from build123d import *

# Parameters (mm, degrees)
F1_DEPTH       = 35
F2_SIZE        = 1
F4_D           = 2.5
F4_DEPTH       = 8
F4_TIP         = 0.7510757738
F6_D           = 4.5
F6_CBORE_D     = 8
F6_CBORE_DEPTH = 5
F8_D           = 3.3
F8_DEPTH       = 12
F8_TIP         = 0.9914200214


with BuildPart() as f1:
    # F0 (on Top) → F1 (new body, symmetric)
    with BuildSketch(Plane.XY):
        Polygon((4, 17), (5, 17), (5, 19), (-5, 19), (-5, -19), (5, -19), (5, -17), (4, -17), (4, 0), align=None)
    extrude(amount=F1_DEPTH, both=True)

    # F2
    f2_edges = [f1.edges().sort_by_distance(p)[0] for p in [
        (-5, 19, 0),
        (5, 19, 0),
        (-5, -19, 0),
        (5, -19, 0),
    ]]
    chamfer(f2_edges, length=F2_SIZE)

    # F4
    with Locations(Plane.XY.offset(35)):
        with Locations((0, 13), (0, -13)):
            Hole(F4_D / 2, depth=F4_DEPTH)
            with Locations((0, 0, -(F4_DEPTH + F4_TIP / 2))):  # 118° drill point
                Cone(0, F4_D / 2, F4_TIP, mode=Mode.SUBTRACT)

    # F6 (through all)
    with Locations(Plane(origin=(-5, 0, 0), x_dir=(0, -1, 0), z_dir=(-1, 0, 0))):
        with Locations((-13, 8), (13, 8), (13, -18), (-13, -18)):
            CounterBoreHole(F6_D / 2, F6_CBORE_D / 2, F6_CBORE_DEPTH)

    # F8
    with Locations(Plane(origin=(0, 0, -35), x_dir=(1, 0, 0), z_dir=(0, 0, -1))):
        with Locations((0, 13), (0, 0), (0, -13)):
            Hole(F8_D / 2, depth=F8_DEPTH)
            with Locations((0, 0, -(F8_DEPTH + F8_TIP / 2))):  # 118° drill point
                Cone(0, F8_D / 2, F8_TIP, mode=Mode.SUBTRACT)


solid = f1.part
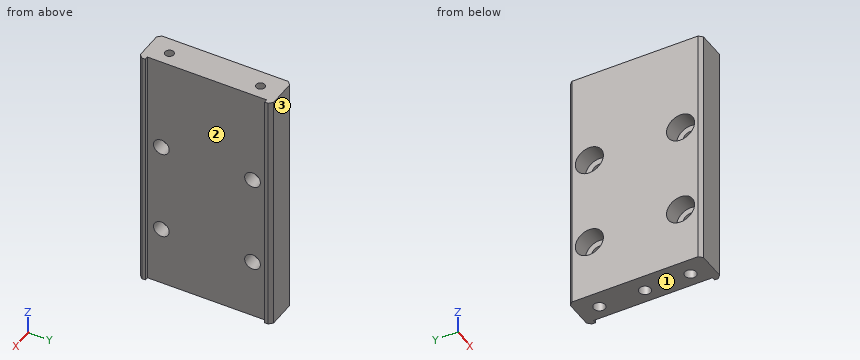
For this review, take the finished solid that the model builds, in its own axes (mm). Face numbers are marked on the shaded views. Round coordinates to 2 decimals unless told otherwise and drop trailing zeros. Write each loop counter-clockwise with the first axis right and the second up, starting at its lowest first coordinate (ties: lowest second). Pieces come first, ordered by that corner, then holes. Notation, with made-up numbers: (15.5, 71) - (72.5, 71) arc R7 cw to (72.5, 78) - close; hole circle Ø9 at (-37.75, 1). An arc over 180 degrees is marked (long way). Use a Markdown table: item, result.
Q1. We need section B-B (z = -29). Give the boundary of the cut face in (x, y), plus the area to 3 significant figures.
Derived:
| item | result |
|---|---|
| outline | (-5, -18) - (-4, -19) - (4, -19) - (5, -18) - (5, -17) - (4, -17) - (4, 17) - (5, 17) - (5, 18) - (4, 19) - (-4, 19) - (-5, 18) - close; hole circle Ø3.3 at (0, -13); hole circle Ø3.3 at (0, 0); hole circle Ø3.3 at (0, 13) |
| area | 318 mm2 |
Q2. Clearance check with flat-ended pins moving along their axes: pin 1 (7 mm diameter, centred on y = 13, z = -18, fed in from -X); pin 2 (1 mm diameter, centred on y = -11.5, z = -23, fed in from +X); pin 3 (1.5 mm diameter, centred on x = 0, y = -13, fed in from -Z); pin 4 (2.5 mm diameter, centred on y = 13, z = -18, fed in from -X). State where each tip first meets the part, or that it passes through.
Derived:
| item | result |
|---|---|
| pin 1 | stops at x = 0 |
| pin 2 | stops at x = 4 |
| pin 3 | stops at z = -22.46 |
| pin 4 | passes through |
Q3. We need section D-D (y = 6.5). Give the boundary of the cut face in (x, z), plus the area to 3 significant figures.
Derived:
| item | result |
|---|---|
| outline | (-5, -35) - (4, -35) - (4, 35) - (-5, 35) - close |
| area | 630 mm2 |
Q4. We need section A-A (z = 8). Give the boundary of the cut face in (x, y), plus the area to 3 significant figures.
Derived:
| item | result |
|---|---|
| outline | (-5, -18) - (-4, -19) - (4, -19) - (5, -18) - (5, -17) - (4, -17) - (4, -15.25) - (0, -15.25) - (0, -17) - (-5, -17) - close; (-5, -9) - (0, -9) - (0, -10.75) - (4, -10.75) - (4, 10.75) - (0, 10.75) - (0, 9) - (-5, 9) - close; (-5, 17) - (0, 17) - (0, 15.25) - (4, 15.25) - (4, 17) - (5, 17) - (5, 18) - (4, 19) - (-4, 19) - (-5, 18) - close |
| area | 228 mm2 |
Q5. The part is to be moulded in two halves that separate along Y. For the marked faces 1, 2 and 3, say which applies: pulls with the +Y half, pulls with the -Y half, needs draft (parallel to the pull), parting line crosses it, or undercut.
Derived:
| item | result |
|---|---|
| face 1 | needs draft |
| face 2 | undercut |
| face 3 | pulls with the +Y half |
Q6. We need section C-C (y = 16). Give the boundary of the cut face in (x, z), plus the area to 3 significant figures.
Derived:
| item | result |
|---|---|
| outline | (-5, -35) - (4, -35) - (4, 35) - (-5, 35) - (-5, 10.65) - (0, 10.65) - (0, 5.35) - (-5, 5.35) - (-5, -15.35) - (0, -15.35) - (0, -20.65) - (-5, -20.65) - close |
| area | 577 mm2 |
Q7. Wall thickness on line 1 along Y through (x, z) = (0, -28.5); line 2 along Z through (x, y) = (2.4, 13); line 3 along Z through (x, y) = (-2.15, -13): over which ranges is each line inside the solid? List them lowest first.
Derived:
| item | result |
|---|---|
| line 1 | y = -19 to -14.65, -11.35 to -1.65, 1.65 to 11.35, 14.65 to 19 |
| line 2 | z = -35 to -20.25, -15.75 to 5.75, 10.25 to 35 |
| line 3 | z = -35 to -22, -14 to 4, 12 to 35 |
